Autodesk Inventor part; units mm, degrees
ref_plane "YZ Plane" through (0, 0, 0) normal (1, 0, 0) x (0, 1, 0)
ref_plane "XZ Plane" through (0, 0, 0) normal (0, 1, 0) x (-1, 0, 0)
ref_plane "XY Plane" through (0, 0, 0) normal (0, 0, 1) x (1, 0, 0)
sketch "Sketch1" plane through (0, 0, 0) normal (0, 1, 0) x (-1, 0, 0)
  line L0 (0, 0) -> (7.3, 0)
  line L1 (7.3, 0) -> (7.3, -34.6)
  line L2 (7.3, -34.6) -> (0, -34.6)
  line L3 (0, -34.6) -> (0, 0)
  dimension "d0" = 7.3
  dimension "d1" = 34.6
extrude "Extrusion1" add sketch "Sketch1" along normal blind 4
chamfer "Chamfer1" distance 0.4 distance2 1.5 1 edges at (0, 4, -17.3) measured on face at (-2.4333, 4, -11.5333)
chamfer "Chamfer2" distance 0.4 distance2 1.5 1 edges at (0, 0, -17.3) measured on face at (-2.4333, 0, -11.5333)
chamfer "Chamfer3" distance 0.4 distance2 1.5 1 edges at (-7.3, 4, -17.3) measured on face at (-2.7, 4, -11.5333)
chamfer "Chamfer4" distance 0.4 distance2 1.5 1 edges at (-7.3, 0, -17.3) measured on face at (-2.7, 0, -11.5333)
ref_plane "Work Plane1" through (-3.65, 2.5, 0) normal (1, 0, 0) x (0, 0, -1)
hole "Hole1" at (-3.65, 4, -34.6) direction (0, -1, 0) diameter 3 depth 0.2
sketch "Sketch3" plane through (0, 2.5, 0) normal (1, 0, 0) x (0, 0, -1)
  line L0 (34.6, -1) -> (34.6, 0)
  line L1 (34.6, -0.5) -> (0, -0.5) construction
  line L2 (0, -1) -> (0, 0)
  line L3 (2.73, -0.375) -> (3.93, -0.375)
  line L4 (3.93, -0.375) -> (3.93, -0.625)
  line L5 (3.93, -0.625) -> (2.73, -0.625)
  line L6 (2.73, -0.625) -> (2.73, -0.375)
  line L7 (2.73, -0.375) -> (3.93, -0.625) construction
  line L8 (3.93, -0.375) -> (2.73, -0.625) construction
  point P0 (0, -2.5)
  point P1 (17.3, -0.5)
  point P2 (3.33, -0.5)
  dimension "d30" = 13.97
  dimension "d31" = 1.2
  dimension "d32" = 0.25
extrude "Extrusion2" cut sketch "Sketch3" against normal through all
pattern_linear "Rectangular Pattern1" count 12 spacing 2.54 along (0, 0, -1) of "Extrusion2"
sketch "Sketch4" plane through (-7.3, 2.5, -34.6) normal (-1, 0, 0) x (0, 0, 1)
  line L0 (33.385, -0.375) -> (34.235, -0.375)
  line L1 (34.235, -0.375) -> (34.235, -0.625)
  line L2 (34.235, -0.625) -> (33.385, -0.625)
  line L3 (33.385, -0.625) -> (33.385, -0.375)
  line L4 (31.87, -0.375) -> (30.67, -0.375)
  line L5 (30.67, -0.375) -> (31.87, -0.375)
  point P0 (34.6, -2.5)
  point P1 (31.27, -0.375)
  point P2 (33.81, -0.375)
  dimension "d38" = 0.85
  dimension "d39" = 0.25
  dimension "d53" = 2.54
extrude "Extrusion3" cut sketch "Sketch4" against normal through all
ref_plane "Work Plane2" through (0, 1.5, -17.3) normal (0, 0, -1) x (-1, 0, 0)
mirror "Mirror2" about plane through (0, 1.5, -17.3) normal (0, 0, -1) of "Extrusion3"
sketch "Sketch5" plane through (0, 4, 0) normal (0, 1, 0) x (1, 0, 0)
  line L0 (-7.3, 0) -> (-7.3, 34.6)
  line L1 (-7.3, 34.6) -> (-5.8, 34.6) construction
  line L2 (-5.8, 34.6) -> (-5.8, 32.6) construction
  line L3 (-5.8, 32.6) -> (-7.3, 32.6) construction
  line L4 (-7.3, 32.6) -> (-7.3, 34.6) construction
  circle A0 centre (-5.8, 32.6) radius 0.5
  point P0 (0, 0)
  dimension "d58" = 2
  dimension "d59" = 1.5
  dimension "d60" = 1
hole "Hole2" at (-5.8, 4, -32.6) direction (0, -1, 0) diameter 1 depth 0.2
equation "\"d4\" = AtmegaChamfer_D1"
equation "\"d5\" = AtmegaChamfer_D2"
equation "\"d7\" = AtmegaChamfer_D1"
equation "\"d8\" = AtmegaChamfer_D2"
equation "\"d10\" = AtmegaChamfer_D1"
equation "\"d11\" = AtmegaChamfer_D2"
equation "\"d13\" = AtmegaChamfer_D1"
equation "\"d14\" = AtmegaChamfer_D2"
equation "\"d31\" = atmegaPinWidth1"
equation "\"d37\" = atmegaPinSpacing"
equation "\"AtmegaChamfer_D1\" = 0.4"
equation "\"atmegaPinDistance\" = 2.54"
equation "\"Thickness\" = 0.25"
equation "\"BendRadius\" = 0.25"
equation "\"BendReliefWidth\" = 0.25"
equation "\"BendReliefDepth\" = 0.125"
equation "\"CornerReliefSize\" = 1"
equation "\"MinimumRemnant\" = 0.5"
equation "\"TransitionRadius\" = 0.25"
equation "\"JacobiRadiusSize\" = 0.25"
equation "\"GapSize\" = 0.25"
equation "\"atmegaPinThickness\" = 0.3"
equation "\"atmegaPinWidth1\" = 1.2"
equation "\"atmegaPinWidth2\" = 0.5"
equation "\"atmegaEndPinWidth\" = 0.9"
equation "\"atmegaPinBendAngle\" = 80deg"
equation "\"atmegaPinBaseWidth\" = 8"
equation "\"atmegaSeatingPlaneDistance\" = 3.2"
equation "\"d27\" = atmegaPinBaseWidth"
equation "\"d28\" = atmegaPinWidth1"
equation "\"d29\" = 0.25"
equation "\"d40\" = BendReliefWidth"
equation "\"d41\" = BendReliefDepth"
equation "\"d42\" = MinimumRemnant"
equation "\"d43\" = TransitionRadius"
equation "\"d45\" = 90deg"
equation "\"d46\" = BendRadius"
equation "\"d47\" = CornerReliefSize"
equation "\"d48\" = GapSize"
equation "\"d49\" = JacobiRadiusSize"
equation "\"d50\" = Thickness"
equation "\"d51\" = 0"
equation "\"d52\" = atmegaSeatingPlaneDistance"
equation "\"d54\" = 0.5 * atmegaPinWidth2"
equation "\"d56\" = 2.5"
equation "\"d44\" = atmegaPinLenght"
equation "\"Atmega28PinsDistance\" = 13 * atmegaPinSpacing"
equation "\"atmegaPinSpacing\" = 2.54"
properties part number "atmega_mold"
Design review of the part built by this model. Coordinates are the model's own, in mm. A direction names the side the tool comes from. Give positions to 0.01 mm unless a question says otherwise; leave off trailing zeros. Order: outer loops, then holes, each group sorted by start corner. A loop starts at its lowest first (then second) coordinate and runs counter-clockwise, first axis right, second up. Notation, with made-up numbers: (4.5, 46) -> (9.5, 46) arc R19 cw to (9.5, 69) -> close; hole circle Ø1 at (3.5, -33). An arc over 180 degrees is marked (long way). Write item = value, one per line. Start each with the question number.
(1) We need section B-B on z = -25. Write out the cut boundary in (x, y).
(2) We need section D-D on y = 0.45. Write out the cut boundary in (x, z), plus the area to 3 significant figures.
(3) For pin 1 (3 mm diameter, centred on x = -5, z = -19.5, fed in from -Y), flat-tipped, find the tip position at first contact; note if it passes through.
(4) To check wall thickness, follow line 1 along Y through (x, z) = (-5.25, -11) (3 decimals); line 2 along Z through (x, y) = (-5.8, 3.85); line 3 along X through (y, z) = (3.95, -32.6). State the ranges of each line that lie inside material, in increasing order.
(5) Mouldability with a two-part tool opening along X and no side actions: class faces 1 (the face through (0, 2, -17.5)), 2 (the face through (-4, 2.125, -11)), 3 (the face through (-4, 3.8, -34)) as +X half, -X half, draft (parallel to the pull), parting line (faces both ways), or undercut.
(6) We need section A-A on z = -16. Write out the cut boundary in (x, y) (3 decimals), plus the area to 3 significant figures.
(7) For faces 4 (the face through (-4, 2.125, -3)), 5 (the face through (-4, 0, -17)), list the 3-axis set-ups (+Z, -Z, +X, -X, +Y, -Y) from which the entire face can be reached by the end or side of a thin tool; tool diameter is ignored.
(8) We need section C-C on x = -5.8. State how many separate pieces and enclosed holes the cut face has, plus the area to 3 significant figures.
Numbers:
q1.outline = (-7.3, 1.5) -> (-6.9, 0) -> (-0.4, 0) -> (0, 1.5) -> (0, 2.5) -> (-0.4, 4) -> (-6.9, 4) -> (-7.3, 2.5) -> close
q2.outline = (-7.02, -34.6) -> (-0.28, -34.6) -> (-0.28, 0) -> (-7.02, 0) -> close
q2.area = 233 mm^2
q3.pin_1 = 0
q4.line_1 = 0 to 1.875, 2.125 to 4
q4.line_2 = -34.6 to -33.1, -32.1 to 0
q4.line_3 = -6.91 to -6.3, -5.3 to -0.39
q5.face_1 = +X half
q5.face_2 = draft
q5.face_3 = undercut
q6.outline = (-7.3, 1.5) -> (-6.9, 0) -> (-0.4, 0) -> (0, 1.5) -> (0, 1.875) -> (-7.3, 1.875) -> close; (-7.3, 2.125) -> (0, 2.125) -> (0, 2.5) -> (-0.4, 4) -> (-6.9, 4) -> (-7.3, 2.5) -> close
q6.area = 26.2 mm^2
q7.face_4 = +X, -X
q7.face_5 = +Z, -Z, +X, -X, -Y
q8.separate_pieces = 1
q8.enclosed_holes = 14
q8.area = 134 mm^2
